Work out the finished part from the listing and answer in its coordinate system (mm). Face numbers are marked on the shaded views. A direction names the side the tool comes from. Coordinates: 2 decimals unless noted, no trailing zeros. Order: outer loops, then holes, each group sorted by start corner. A loop starts at its lowest first (then second) coordinate and runs counter-clockwise, first axis right, second up. Notation, with made-up numbers: M -28.5,72 L -11.5,72 A25 cw -11.5,92 Z; hole C 11,5 d5. An arc over 180 degrees is marked long. Write item = value, one per line. Start each with the question number.
Q1. Find section C-C on z = 2.25. Give the vertices of the cut face in (x, y).
Q2. A tool of negligible diameter and unlimited length cuts with its end or side. For the marked faces 4 and 5, from which of +Z, -Z, +X, -X, +Y, -Y can it reach the whole face along a straight path? Write none if from no direction.
Q3. Each of these flat-tipped pins is pushed along its axis until it touches: P1, Ø4, axis at x = 0.5, z = -4.5, coming from the -Y side; P2, Ø2, axis at x = -2, z = -11.5, coming from the +Y side; P3, Ø3, axis at x = -0.5, z = -14.5, coming from the +Y side. Where does it stop, or does it pass through?
Q4. Determine the mould class of the marked faces 1, 2 and 3 for opening direction Y: released by +Y, released by -Y, zero draft, split by the parting line, or undercut.
Q5. Straight lines are drawn through the part: line 1 along Z through (x, y) = (4.25, 1.5); line 2 along Z through (x, y) = (-0.25, 1); line 3 along X through (y, z) = (0, -17.25). For each, find the intervals that lie inside material, in ascending order.
Q6. Find section A-A on y = 0. Give the vertices of the cut face in (x, z).
Q7. Find section B-B on z = -1.25. Give the vertices of the cut face in (x, y), and give its area (3 significant figures).
```python
from build123d import *

# Parameters (mm, degrees)
F0_R     = 5
F1_DEPTH = 6
F2_R     = 0.5
F4_DEPTH = 3
F5_R     = 3
F6_DEPTH = 20
F7_SIZE  = 1


with BuildPart() as f1:
    # F0 (on Top) → F1 (new body)
    with BuildSketch(Plane.XY):
        Circle(F0_R)
    extrude(amount=F1_DEPTH)

    # F2
    f2_edges = [f1.edges().sort_by_distance(p)[0] for p in [
        (-5, 0, 6),
    ]]
    fillet(f2_edges, radius=F2_R)

    # F3 (on face) → F4 (cut)
    with BuildSketch(Plane.XY.offset(6)):
        Polygon((2.5, 1.443376), (0, 2.886751), (-2.5, 1.443376), (-2.5, -1.443376), (0, -2.886751), (2.5, -1.443376), align=None)
    extrude(amount=-F4_DEPTH, mode=Mode.SUBTRACT)

    # F5 (on face) → F6 (join)
    with BuildSketch(Plane(origin=(0, 0, 0), x_dir=(1, 0, 0), z_dir=(0, 0, -1))):
        Circle(F5_R)
    extrude(amount=F6_DEPTH)

    # F7
    f7_edges = [f1.edges().sort_by_distance(p)[0] for p in [
        (-3, 0, -20),
    ]]
    chamfer(f7_edges, length=F7_SIZE)


solid = f1.part
```
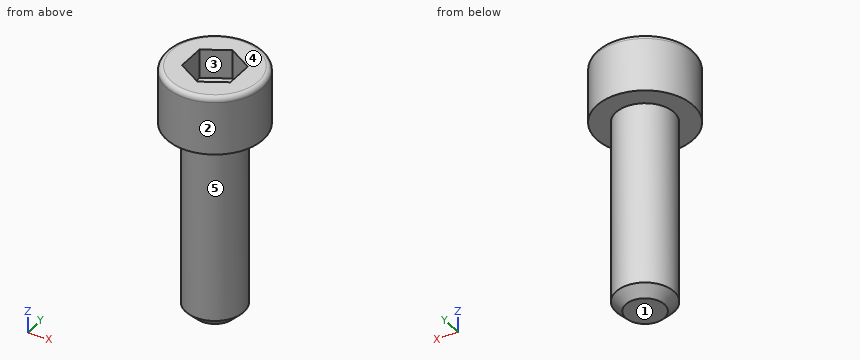
Findings below:
q1.outline = C 0,0 d10
q2.face_4 = +Z, +X, -X, +Y, -Y
q2.face_5 = -Z
q3.P1 = -3
q3.P2 = 2.83
q3.P3 = 3
q4.face_1 = zero draft
q4.face_2 = split by the parting line
q4.face_3 = undercut
q5.line_1 = 0 to 6
q5.line_2 = -20 to 3
q5.line_3 = -3 to 3
q6.outline = M -5,0 L -3,0 L -3,-19 L -2,-20 L 2,-20 L 3,-19 L 3,0 L 5,0 L 5,5.5 A0.5 ccw 4.5,6 L 2.5,6 L 2.5,3 L -2.5,3 L -2.5,6 L -4.5,6 A0.5 ccw -5,5.5 Z
q7.outline = C 0,0 d6
q7.area = 28.3 mm^2
